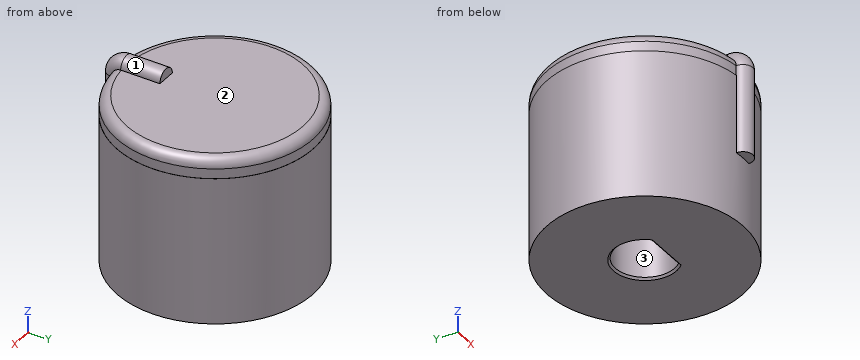
from build123d import *

# Parameters (mm, degrees)
F0_R     = 10
F1_DEPTH = 15
F2_R     = 9.9864299767
F9_DEPTH = 2
F3_R     = 1
F4_SIZE  = 0.2
F7_R     = 1


with BuildPart() as f1:
    # F0 (on Top) → F1 (new body)
    with BuildSketch(Plane.XY):
        Circle(F0_R)
        with BuildLine():
            ThreePointArc((-2.2405356502, -2.01), (0, 3.01), (2.2405356502, -2.01))
            Line((2.2405356502, -2.01), (-2.2405356502, -2.01))
        make_face(mode=Mode.SUBTRACT)
    extrude(amount=F1_DEPTH)

    # F2 (on face) → F9 (join)
    with BuildSketch(Plane.XY.offset(15)):
        Circle(F2_R)
        with BuildLine():
            Line((2.2405356502, -2.01), (-2.2405356502, -2.01))
            ThreePointArc((-2.2405356502, -2.01), (0, 3.01), (2.2405356502, -2.01))
        make_face(mode=Mode.SUBTRACT)
        Circle(F2_R)
    extrude(amount=F9_DEPTH)

    # F3
    f3_edges = [f1.edges().sort_by_distance(p)[0] for p in [
        (-9.98643, 0, 17),
    ]]
    fillet(f3_edges, radius=F3_R)

    # F4
    f4_edges = [f1.edges().sort_by_distance(p)[0] for p in [
        (0, 3.01, 0),
        (0, -2.01, 0),
    ]]
    chamfer(f4_edges, length=F4_SIZE)

    # F8: sweep along a path in F5
    with BuildLine(Plane.YZ) as f8_path:
        Line((-9.9864299767, 7), (-9.9864299767, 16))
        ThreePointArc((-9.9864299767, 16), (-9.6935367579, 16.7071067812), (-8.9864299767, 17))
        Line((-8.9864299767, 17), (-4.9864299767, 17))
    # F7 (on line) → F8 (sweep)
    with BuildSketch(Plane(origin=(0, 0, 7), x_dir=(1, 0, 0), z_dir=(0, 0, -1))):
        with Locations((0, 9.9864299767)):
            Circle(F7_R)
    sweep(path=f8_path.line)


solid = f1.part
CAD build for the part. Positions are in the model's coordinates, mm. Face numbers are marked on the shaded views. Round coordinates to 2 decimals unless told otherwise and drop trailing zeros. Order: outer loops, then holes, each group sorted by start corner. A loop starts at its lowest first (then second) coordinate and runs counter-clockwise, first axis right, second up. Notation, with made-up numbers: (84.25, -31.75) -> (109.25, -31.75) arc R16 ccw to (109.25, -22.75) -> close; hole circle Ø8 at (83.25, 26.5). An arc over 180 degrees is marked (long way). Write item = value, one per line. Start each with the question number.
(1) Cut at D-D, the plane z = 13. List the corners of the cut face in (x, y).
(2) Probe line 1 (X direction, y = 0, z = 5.5); line 2 (Z direction, x = 2.5, y = 2.5); line 3 (Y direction, x = 2, z = 11.75). List the from-to ranges inside material, lowest first. Write a range as [from, to].
(3) Cut at C-C, the plane z = 15.5. List the corners of the cut face in (x, y), then the cut area to 3 significant figures.
(4) Pull direction X, two halves, no side cores. Call the marked faces 1, 2 and 3: released by +X, released by -X, zero draft, split by the parting line, or undercut.
(5) Cut at A-A, the plane z = 5.5. List the corners of the cut face in (x, y), then the cut area to 3 significant figures.
(6) Pin check, flat tips, straight feed: P1, Ø6, axis at x = -1.5, y = -3, coming from the -Z side; P2, Ø10, axis at x = 4, y = 3, coming from the +Z side; P3, Ø1.3, axis at x = 1, z = 4, coming from the +Y side; P4, Ø5, axis at x = 8, z = 3.5, coming from the -Y side. Stop position of each tip, or through.
Model answer:
q1.outline = (-1, -9.95) arc R1 ccw (long way) to (1, -9.95) arc R10 ccw (long way) to start; hole (-2.24, -2.01) -> (2.24, -2.01) arc R3.01 ccw (long way) to start
q2.line_1 = [-10, -3.01], [3.01, 10]
q2.line_2 = [0, 17]
q2.line_3 = [-9.8, -2.01], [2.25, 9.8]
q3.outline = (-1, -9.94) arc R1 ccw (long way) to (1, -9.94) arc R9.99 ccw (long way) to start
q3.area = 315 mm2
q4.face_1 = split by the parting line
q4.face_2 = zero draft
q4.face_3 = undercut
q5.outline = circle Ø20 at (0, 0); hole (-2.24, -2.01) -> (2.24, -2.01) arc R3.01 ccw (long way) to start
q5.area = 289 mm2
q6.P1 = 0
q6.P2 = 17
q6.P3 = 9.99
q6.P4 = -8.35
